Build history of the part. All positions in model axes, mm. A direction names the side the tool comes from. Give positions to 0.01 mm unless a question says otherwise; leave off trailing zeros. Loops run counter-clockwise (first coordinate to the right, second up) from the corner with the lowest first, then second, coordinate; pieces in that order, holes last. Notation, with made-up numbers: (31, 14.25) -> (42, 14.25) arc R17 ccw to (42, 37.25) -> close; hole circle Ø4 at (11.5, 0.5). An arc over 180 degrees is marked (long way). Answer as a JSON object with one key per item and string values. Group by question number.
Q1. Band-saw the part on B-B, the plane x = 0. Write the cut outline in (y, z), plus the area to 3 significant figures.
Q2. Band-saw the part on A-A, the plane y = 29. Write the cut outline in (x, z).
Q3. Two-plate mould, pull along X, no slides. Class faces 4 (the flat face through (0, -36.398, 0)), 5 (the flat face through (3.48, -0.66, -1.97)), 6 (the flat face through (1, 47.498, -2)): pulls with the +X half, pulls with the -X half, needs draft (parallel to the pull), parting line crosses it, or undercut.
Q4. Wall check: probe 1 along X at (y, z) = (45.75, 0); probe 2 along Y at (x, z) = (0, 1.75); probe 3 along X at (y, z) = (40, -1.5). Give the ranges that are in metal, low to high. Write a range as from..to.
Q5. Tool access for faces 1 (the cylindrical face through (-2, -42, 0)), 2 (the cylindrical face through (2, 42, 0)), 3 (the flat face through (1, -47.498, -2)): list every direction of +Z, -Z, +X, -X, +Y, -Y with a clear straight run to the whole face (end or side of a thin tool).
Q6. Drop a flat-ended pin along its axis: pin 1 (2.5 mm diameter, centred on x = 0, z = 0, fed in from +Y). Give the stop position or say it passes through.
from build123d import *

# Parameters (mm, degrees)
BOSS_EXTRUDE1_DEPTH      = 47.498
BOSS_EXTRUDE1_DEPTH_BACK = 47.498
SKETCH3_R                = 2
CUT_EXTRUDE1_DEPTH       = 11.1
CUT_EXTRUDE2_START       = -10
SKETCH2_R                = 2
CUT_EXTRUDE2_DEPTH       = 10


with BuildPart() as part:
    # Sketch1 → Boss-Extrude1 (new, two sides: drawn at the far end of the back side and taken through both)
    with BuildSketch(Plane(origin=(0, 0, 0), x_dir=(1, 0, 0), z_dir=(0, 1, 0)).offset(-BOSS_EXTRUDE1_DEPTH_BACK)):
        Polygon((2.309401077, 4), (-2.309401077, 4), (-4.618802154, 0), (-2.309401077, -4), (2.309401077, -4), (4.618802154, 0), align=None)
    extrude(amount=BOSS_EXTRUDE1_DEPTH + BOSS_EXTRUDE1_DEPTH_BACK)

    # Sketch3 → Cut-Extrude1 (cut)
    with BuildSketch(Plane.XZ.offset(47.498)):
        with Locations(Location((0, 0, 0), (0, 0, 270))):
            Circle(SKETCH3_R)
    extrude(amount=-CUT_EXTRUDE1_DEPTH, mode=Mode.SUBTRACT)

    # Sketch2 → Cut-Extrude2 (cut)
    with BuildSketch(Plane(origin=(0, 47.498, 0), x_dir=(1, 0, 0), z_dir=(0, 1, 0)).offset(CUT_EXTRUDE2_START)):
        with Locations(Location((0, 0, 0), (0, 0, 90))):
            Circle(SKETCH2_R)
    extrude(amount=CUT_EXTRUDE2_DEPTH, mode=Mode.SUBTRACT)


solid = part.part
Worked answers:
{
 "1": {"outline": "(-47.5, -4) -> (47.5, -4) -> (47.5, -2) -> (37.5, -2) -> (37.5, 2) -> (47.5, 2) -> (47.5, 4) -> (-47.5, 4) -> (-47.5, 2) -> (-36.4, 2) -> (-36.4, -2) -> (-47.5, -2) -> close", "area": "676 mm2"},
 "2": {"outline": "(-4.62, 0) -> (-2.31, -4) -> (2.31, -4) -> (4.62, 0) -> (2.31, 4) -> (-2.31, 4) -> close"},
 "3": {"face 4": "undercut", "face 5": "pulls with the +X half", "face 6": "needs draft"},
 "4": {"probe 1": "-4.62..-2, 2..4.62", "probe 2": "-36.4..37.5", "probe 3": "-3.75..-1.32, 1.32..3.75"},
 "5": {"face 1": "-Y", "face 2": "+Y", "face 3": "+Z, -Z, +X, -X, -Y"},
 "6": {"pin 1": "y = 37.5"}
}
